Geometry check sheet. Reference: the model listing, model coordinates, mm. A direction names the side the tool comes from. Give positions to 0.01 mm unless a question says otherwise; leave off trailing zeros. Write each loop counter-clockwise with the first axis right and the second up, starting at its lowest first coordinate (ties: lowest second). Pieces come first, ordered by that corner, then holes. Notation, with made-up numbers: (39, -25) -> (44, -25) arc R31 ccw to (44, 12) -> close; hole circle Ø4 at (-23, 28.25). An arc over 180 degrees is marked (long way). Use a Markdown table: item, result. Add a question column.
from build123d import *

# Parameters (mm, degrees)
SKETCH1_R               = 6.4
BOSS_EXTRUDE1_DEPTH     = 5.6
HORN_START              = -2
HORN_DEPTH              = 2
SKETCH4_R               = 1.4
CUT_EXTRUDE1_DEPTH      = 26.681786257
SKETCH5_R               = 0.75
CUT_EXTRUDE2_DEPTH      = 26.681786257
LPATTERN1_COUNT         = 4
LPATTERN1_PITCH         = 3
MIRROR1_COPY_1_SKETCH_R = 0.75
MIRROR1_COPY_1_DEPTH    = 26.681786257
MIRROR1_COPY_2_SKETCH_R = 0.75
MIRROR1_COPY_2_DEPTH    = 26.681786257
MIRROR1_COPY_3_SKETCH_R = 0.75
MIRROR1_COPY_3_DEPTH    = 26.681786257
CUT_EXTRUDE4_DEPTH      = 3
CIRPATTERN2_COUNT       = 26
SKETCH9_R               = 2.6
CUT_EXTRUDE5_DEPTH      = 3
SKETCH10_R              = 6.4
SKETCH10_R_2            = 4.25
CUT_EXTRUDE6_DEPTH      = 3.6
SKETCH12_R              = 4.45
CUT_EXTRUDE7_DEPTH      = 1
SKETCH13_R              = 3.45
SKETCH13_R_2            = 2.95
BOSS_EXTRUDE6_DEPTH     = 1
SKETCH14_R              = 3.45
SKETCH14_R_2            = 2.95
BOSS_EXTRUDE7_DEPTH     = 0.35


with BuildPart() as part:
    # Sketch1 → Boss-Extrude1 (new body)
    with BuildSketch(Plane(origin=(0, 0, 0), x_dir=(1, 0, 0), z_dir=(0, 1, 0))):
        with Locations(Location((0, 0, 0), (0, 0, 270))):
            Circle(SKETCH1_R)
    extrude(amount=BOSS_EXTRUDE1_DEPTH)

    # Sketch2 → horn (add)
    with BuildSketch(Plane(origin=(0, 5.6, 0), x_dir=(1, 0, 0), z_dir=(0, 1, 0)).offset(HORN_START)):
        with BuildLine():
            Line((-2.609740545, 22.043082174), (-6.271723477, 1.27494495))
            ThreePointArc((-6.271723477, 1.27494495), (0, 6.4), (6.271723477, 1.27494495))
            Line((6.271723477, 1.27494495), (2.609740545, 22.043082174))
            ThreePointArc((2.609740545, 22.043082174), (0, 24.232914504), (-2.609740545, 22.043082174))
        make_face()
    horn = extrude(amount=HORN_DEPTH)

    # Sketch4 → Cut-Extrude1 (cut, through all)
    with BuildSketch(Plane(origin=(0, 5.6, 0), x_dir=(-1, 0, 0), z_dir=(0, -1, 0))):
        with Locations(Location((0, 0, 0), (0, 0, 90))):
            Circle(SKETCH4_R)
    extrude(amount=CUT_EXTRUDE1_DEPTH, mode=Mode.SUBTRACT)

    # Sketch5 → Cut-Extrude2 (cut, through all)
    with BuildSketch(Plane(origin=(0, 0, 0), x_dir=(-1, 0, 0), z_dir=(0, -1, 0))):
        with Locations(Location((0, 20.882914504, 0), (0, 0, 90))):
            Circle(SKETCH5_R)
    cut_extrude2 = extrude(amount=-CUT_EXTRUDE2_DEPTH, mode=Mode.SUBTRACT)

    # LPattern1: Cut-Extrude2 ×4
    with Locations(*[(0, 0, i * LPATTERN1_PITCH) for i in range(1, LPATTERN1_COUNT)]):
        add(cut_extrude2, mode=Mode.SUBTRACT)

    # Mirror1: horn, Cut-Extrude2 across plane
    add(horn.mirror(Plane.XY))
    add(cut_extrude2.mirror(Plane.XY), mode=Mode.SUBTRACT)

    # Mirror1 copy 1 sketch → Mirror1 copy 1 (cut, through all)
    with BuildSketch(Plane(origin=(0, 0, -3), x_dir=(-1, 0, 0), z_dir=(0, -1, 0))):
        with Locations((0, -20.882914504)):
            Circle(MIRROR1_COPY_1_SKETCH_R)
    extrude(amount=-MIRROR1_COPY_1_DEPTH, mode=Mode.SUBTRACT)

    # Mirror1 copy 2 sketch → Mirror1 copy 2 (cut, through all)
    with BuildSketch(Plane(origin=(0, 0, -6), x_dir=(-1, 0, 0), z_dir=(0, -1, 0))):
        with Locations((0, -20.882914504)):
            Circle(MIRROR1_COPY_2_SKETCH_R)
    extrude(amount=-MIRROR1_COPY_2_DEPTH, mode=Mode.SUBTRACT)

    # Mirror1 copy 3 sketch → Mirror1 copy 3 (cut, through all)
    with BuildSketch(Plane(origin=(0, 0, -9), x_dir=(-1, 0, 0), z_dir=(0, -1, 0))):
        with Locations((0, -20.882914504)):
            Circle(MIRROR1_COPY_3_SKETCH_R)
    extrude(amount=-MIRROR1_COPY_3_DEPTH, mode=Mode.SUBTRACT)

    # Sketch8 → Cut-Extrude4 (cut)
    with BuildSketch(Plane(origin=(0, 0, 0), x_dir=(-1, 0, 0), z_dir=(0, -1, 0))):
        with BuildLine():
            Line((0, -2.9), (0.262912611, -2.586672952))
            ThreePointArc((0.262912611, -2.586672952), (0, -2.6), (-0.262912611, -2.586672952))
            Line((-0.262912611, -2.586672952), (0, -2.9))
        make_face()
    cut_extrude4 = extrude(amount=-CUT_EXTRUDE4_DEPTH, mode=Mode.SUBTRACT)

    # CirPattern2: Cut-Extrude4 ×26 about axis
    cirpattern2_axis = Axis((0, 0, 0), (0, 1, 0))
    for i in range(1, CIRPATTERN2_COUNT):
        add(cut_extrude4.rotate(cirpattern2_axis, i * 360 / CIRPATTERN2_COUNT), mode=Mode.SUBTRACT)

    # Sketch9 → Cut-Extrude5 (cut)
    with BuildSketch(Plane(origin=(0, 0, 0), x_dir=(-1, 0, 0), z_dir=(0, -1, 0))):
        Circle(SKETCH9_R)
    extrude(amount=-CUT_EXTRUDE5_DEPTH, mode=Mode.SUBTRACT)

    # Sketch10 → Cut-Extrude6 (cut)
    with BuildSketch(Plane(origin=(0, 0, 0), x_dir=(-1, 0, 0), z_dir=(0, -1, 0))):
        Circle(SKETCH10_R)
        with Locations(Location((0, 0, 0), (0, 0, 90))):
            Circle(SKETCH10_R_2, mode=Mode.SUBTRACT)
    extrude(amount=-CUT_EXTRUDE6_DEPTH, mode=Mode.SUBTRACT)

    # Sketch12 → Cut-Extrude7 (cut)
    with BuildSketch(Plane(origin=(0, 5.6, 0), x_dir=(1, 0, 0), z_dir=(0, 1, 0))):
        with Locations(Location((0, 0, 0), (0, 0, 270))):
            Circle(SKETCH12_R)
    extrude(amount=-CUT_EXTRUDE7_DEPTH, mode=Mode.SUBTRACT)

    # Sketch13 → Boss-Extrude6 (add)
    with BuildSketch(Plane(origin=(0, 4.6, 0), x_dir=(1, 0, 0), z_dir=(0, 1, 0))):
        with Locations(Location((0, 0, 0), (0, 0, 90))):
            Circle(SKETCH13_R)
        with Locations(Location((0, 0, 0), (0, 0, 90))):
            Circle(SKETCH13_R_2, mode=Mode.SUBTRACT)
    extrude(amount=BOSS_EXTRUDE6_DEPTH)

    # Sketch14 → Boss-Extrude7 (add)
    with BuildSketch(Plane(origin=(0, 5.6, 0), x_dir=(1, 0, 0), z_dir=(0, 1, 0))):
        with Locations(Location((0, 0, 0), (0, 0, 90))):
            Circle(SKETCH14_R)
        with Locations(Location((0, 0, 0), (0, 0, 90))):
            Circle(SKETCH14_R_2, mode=Mode.SUBTRACT)
    extrude(amount=BOSS_EXTRUDE7_DEPTH)


solid = part.part
1) Sectioned sample at A-A, the plane z = -15. Enter the section's corners in (x, y).
2) Sectioned sample at B-B, the plane y = 5.05. Count the separate pieces of the cut face and the enclosed holes in it, and give its area (3 significant figures).
3) Draft check along Z on faces 3 (the face through (2.88, 5.27, 0.64)), 4 (the face through (-3, 0, 0)), 5 (the face through (6.4, 4.6, 0)). Enter one of: +Z half, -Z half, draft (parallel to the pull), parting line (faces both ways), or undercut.
4) Tool access check on faces 1 (the face through (3.01, 5.11, -3.28)), 2 (the face through (0.052, 4.586, -24.232)). Record the directions out of +Z, -Z, +X, -X, +Y, -Y that give a thin tool (end or side, any length) a straight path to the whole face; none if there is none.
5) Gauge pin test, flat ends, axial feed: P1, Ø5, axis at x = 3.5, z = 8.5, coming from the -Y side; P2, Ø3, axis at x = 1.5, y = 5, coming from the -Z side; P3, Ø1, axis at y = 4, z = 7, coming from the -X side; P4, Ø2, axis at x = 0, z = 17.88, coming from the +Y side. Record the tip position at first contact, or that the pin passes through.
6) Sectioned sample at D-D, the plane z = -9. Enter the section's corners in (x, y), and give its area (3 significant figures).
7) Material ranges on probe 1 along Y at (x, z) = (4.5, 4); probe 2 along X at (y, z) = (5.7, 1.5); probe 3 along Z at (x, y) = (0.5, 0.5), recorded low to high. Write a range as [from, to].
8) Sectioned sample at C-C, the plane x = -5.5. Enter the section's corners in (y, z).
Check values:
| question | item | result |
|---|---|---|
| 1 | outline | (-3.85, 3.6) -> (-0.74, 3.6) -> (-0.74, 5.6) -> (-3.85, 5.6) -> close; (0.74, 3.6) -> (3.85, 3.6) -> (3.85, 5.6) -> (0.74, 5.6) -> close |
| 2 | separate pieces | 2 |
| 2 | enclosed holes | 10 |
| 2 | area | 352 mm² |
| 3 | face 3 | undercut |
| 3 | face 4 | draft |
| 3 | face 5 | parting line |
| 4 | face 1 | +Y |
| 4 | face 2 | -Z, +Y, -Y |
| 5 | P1 | y = 3.6 |
| 5 | P2 | z = -24.23 |
| 5 | P3 | x = -5.35 |
| 5 | P4 | y = 5.6 |
| 6 | outline | (-4.91, 3.6) -> (4.91, 3.6) -> (4.91, 5.6) -> (-4.91, 5.6) -> close |
| 6 | area | 19.6 mm² |
| 7 | probe 1 | [3.6, 5.6] |
| 7 | probe 2 | [-3.11, -2.54], [2.54, 3.11] |
| 7 | probe 3 | [-4.22, -2.67], [2.67, 4.22] |
| 8 | outline | (3.6, -5.65) -> (5.6, -5.65) -> (5.6, 5.65) -> (3.6, 5.65) -> close |
